Design review of the part built by this model. Coordinates are the model's own, in mm. Face numbers are marked on the shaded views. A direction names the side the tool comes from. Give positions to 0.01 mm unless a question says otherwise; leave off trailing zeros. Write each loop counter-clockwise with the first axis right and the second up, starting at its lowest first coordinate (ties: lowest second). Pieces come first, ordered by that corner, then holes. Notation, with made-up numbers: (15.25, -6.75) -> (48.25, -6.75) arc R20 ccw to (48.25, 31.25) -> close; hole circle Ø10 at (54, 8.25). An arc over 180 degrees is marked (long way). Put each result on its own line as item: value. Start each with the question number.
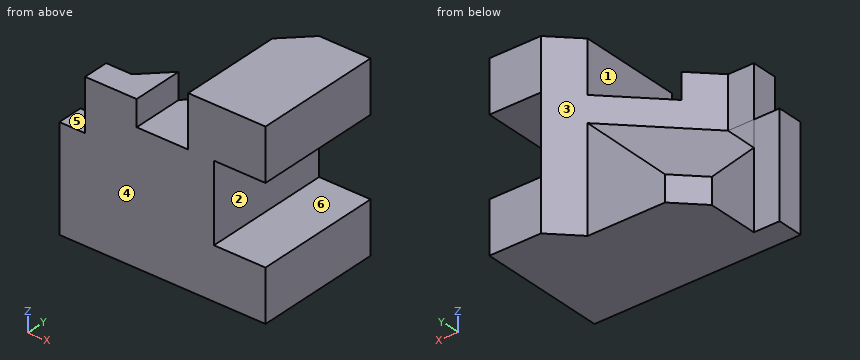
from build123d import *

# Parameters (mm, degrees)
BOSS_EXTRUDE1_DEPTH     = 5
CUT_EXTRUDE1_DEPTH      = 5
CUT_EXTRUDE1_DEPTH_BACK = 2
CUT_EXTRUDE3_DEPTH      = 5
SKETCH5_W               = 4
SKETCH5_H               = 3
CUT_EXTRUDE4_DEPTH      = 1
CUT_EXTRUDE5_DEPTH      = 1
CUT_EXTRUDE6_DEPTH      = 1


with BuildPart() as part:
    # Sketch1 → Boss-Extrude1 (new body)
    with BuildSketch(Plane(origin=(0, 0, 0), x_dir=(1, 0, 0), z_dir=(0, 1, 0))):
        Polygon((0, 0), (0, -2), (-2, -2), (-2, -5), (0, -5), (0, -7), (-3, -7), (-3, -5), (-5, -5), (-5, -6), (-7, -6), (-7, -4), (-8, -4), (-8, 0), align=None)
    extrude(amount=BOSS_EXTRUDE1_DEPTH)

    # Sketch2 → Cut-Extrude1 (cut, two sides)
    with BuildSketch(Plane.XY.offset(6)) as cut_extrude1_sk:
        Polygon((-8, 1), (-6, 1), (-2, 5), (-8, 5), align=None)
    extrude(amount=CUT_EXTRUDE1_DEPTH, mode=Mode.SUBTRACT)
    extrude(cut_extrude1_sk.sketch, amount=-CUT_EXTRUDE1_DEPTH_BACK, mode=Mode.SUBTRACT)

    # Sketch3 → Cut-Extrude3 (cut)
    with BuildSketch(Plane.XY.offset(4)):
        Polygon((-2, 5), (-3, 5), (-8, 5), (-8, 4), (-3, 4), align=None)
    extrude(amount=-CUT_EXTRUDE3_DEPTH, mode=Mode.SUBTRACT)

    # Sketch5 → Cut-Extrude4 (cut)
    with BuildSketch(Plane.ZY.offset(8)):
        with Locations((2, 2.5)):
            Rectangle(SKETCH5_W, SKETCH5_H)
    extrude(amount=-CUT_EXTRUDE4_DEPTH, mode=Mode.SUBTRACT)

    # Sketch7 → Cut-Extrude5 (cut)
    with BuildSketch(Plane(origin=(0, 0, 0), x_dir=(-1, 0, 0), z_dir=(0, 0, -1))):
        Polygon((6, 4), (7, 3), (7, 4), align=None)
    extrude(amount=-CUT_EXTRUDE5_DEPTH, mode=Mode.SUBTRACT)

    # 3DSketch1 → Cut-Extrude6 (cut, along a direction that is not the sketch's normal)
    with BuildSketch(Plane(origin=(-7, 1, 3), x_dir=(0.7844645405527364, 0.588348405414552, 0.19611613513818382), z_dir=(-0.5773502691896255, 0.577350269189626, 0.5773502691896261))):
        Polygon((0, 0), (0.784464541, 2.717464882), (2.157277487, 3.057147992), (5.099019514, 0), (0.980580676, -1.019049331), align=None)
    extrude(amount=CUT_EXTRUDE6_DEPTH, dir=(-1, 0, 0), mode=Mode.SUBTRACT)


with BuildPart() as body_2:
    # of the pieces the cut leaves, the one that is kept (cut_extrude6_keep)
    add(part.part.solids().sort_by_distance((0, 0, 0))[0])


solid = body_2.part
Q1. Machinability: for the marked faces 1, 2 and 3, which of the approach directions +Z, -Z, +X, -X, +Y, -Y give a long, thin tool a straight path to every point of the face, cutting with its end or side? Answer none if there is none.
Q2. For pin 1 (3 mm diameter, centred on x = -3, z = 6.5, fed in from -Y); pin 2 (1.6 mm diameter, centred on x = -6, y = 1.5, fed in from +Z); pin 3 (2 mm diameter, centred on y = 2.5, z = 1.5, fed in from -X); pin 4 (1 mm diameter, centred on x = -5.5, z = 4.5, fed in from +Y), all flat-tipped, find the tip position at first contact; note any pin that passes through.
Q3. Take a section at A-A on x = -1. Give the boundary of the cut face in (y, z), then the cut area to 3 significant figures.
Q4. Take a section at C-C on y = 1.85. Give the boundary of the cut face in (x, z), then the cut area to 3 significant figures.
Q5. Mouldability with a two-part tool opening along Z and no side actions: class the marked faces 4, 5 and 6 as +Z half, -Z half, draft (parallel to the pull), parting line (faces both ways), or undercut.
Q6. To check wall thickness, follow probe 1 along Z at (x, y) = (-1, 3); probe 2 along X at (y, z) = (0.4, 2.75); probe 3 along X at (y, z) = (2.3, 5.75). State the ranges of each line that lie inside material, in increasing order. Write a range as from..to.
Q7. Take a section at B-B on z = 5.5. Give the boundary of the cut face in (x, y).
Q8. Take a section at D-D on x = -6.5. Give the boundary of the cut face in (y, z), then the cut area to 3 significant figures.
Result:
1. face 1: +Z, +Y, -Y
1. face 2: +X, +Y, -Y
1. face 3: +Z, -X, +Y
2. pin 1: stops at y = 0
2. pin 2: stops at z = 6
2. pin 3: stops at x = -7
2. pin 4: stops at y = 2
3. outline: (0, 0) -> (5, 0) -> (5, 2) -> (0, 2) -> close; (0, 5) -> (5, 5) -> (5, 7) -> (0, 7) -> close
3. area: 20.0 mm^2
4. outline: (-7, 0) -> (0, 0) -> (0, 2) -> (-2, 2) -> (-2, 5) -> (0, 5) -> (0, 7) -> (-3, 7) -> (-3, 5) -> (-5, 5) -> (-5, 6) -> (-5.15, 6) -> (-5.15, 4) -> (-7, 2.15) -> close
4. area: 31.6 mm^2
5. face 4: draft
5. face 5: +Z half
5. face 6: undercut
6. probe 1: z = 0..2, 5..7
6. probe 2: x = -8..-2
6. probe 3: x = -3..0
7. outline: (-7, 0) -> (-5, 0) -> (-5, 2) -> (-6, 1) -> (-7, 1) -> close; (-3, 0) -> (0, 0) -> (0, 5) -> (-2, 5) -> (-3, 4) -> close
8. outline: (0, 0) -> (3.5, 0) -> (3.5, 1) -> (1, 3.5) -> (1, 6) -> (0, 6) -> close
8. area: 11.6 mm^2
